Can you work these out from the model? Positions are in its coordinate system, mm. A direction names the side the tool comes from. Give positions to 0.01 mm unless a question says otherwise; leave off trailing zeros. Write each loop counter-clockwise with the first axis right and the second up, starting at its lowest first coordinate (ties: lowest second). Pieces come first, ordered by that corner, then holes.
from build123d import *

# Parameters (mm, degrees)
F0_R     = 1.5
F1_DEPTH = 3
F2_R     = 4.5
F3_DEPTH = 5.2
F4_R     = 1.5
F5_DEPTH = 20


with BuildPart() as f1:
    # F0 (on Front) → F1 (new body)
    with BuildSketch(Plane.XZ):
        with BuildLine():
            Line((5.9394528039, 2.640625), (2.9697264019, 9.3203125))
            ThreePointArc((2.9697264019, 9.3203125), (0, 11.25), (-2.9697264019, 9.3203125))
            Line((-2.9697264019, 9.3203125), (-5.9394528039, 2.640625))
            ThreePointArc((-5.9394528039, 2.640625), (0, -6.5), (5.9394528039, 2.640625))
        make_face()
        with Locations((0, 8)):
            Circle(F0_R, mode=Mode.SUBTRACT)
    extrude(amount=-F1_DEPTH)

    # F2 (on face) → F3 (join)
    with BuildSketch(Plane.XZ):
        Circle(F2_R)
    extrude(amount=F3_DEPTH)

    # F4 (on face) → F5 (cut)
    with BuildSketch(Plane.XZ.offset(5.2)):
        Circle(F4_R)
    extrude(amount=-F5_DEPTH, mode=Mode.SUBTRACT)


solid = f1.part
(1) Will these pins go through, and if not, where does the flat tip stop? P1, Ø2, axis at x = 2.5, y = -0.5, coming from the -Z side; P2, Ø3, axis at y = -2.5, z = 7, coming from the +X side (1 decimal); P3, Ø3, axis at y = 0, z = -1.5, coming from the -X side; P4, Ø3, axis at x = 3, y = 2, coming from the +Z side.
Returned:
P1: stops at z = -6.29
P2: passes through
P3: stops at x = -6.5
P4: stops at z = 10.88
(2) Imagine slicing it at B-B, the plane x = 0. Write out the boundary of the cut face in (y, z), plus the area to 4 significant figures.
Returned:
outline: (-5.2, -4.5) - (0, -4.5) - (0, -6.5) - (3, -6.5) - (3, -1.5) - (-5.2, -1.5) - close; (-5.2, 1.5) - (3, 1.5) - (3, 6.5) - (0, 6.5) - (0, 4.5) - (-5.2, 4.5) - close; (0, 9.5) - (3, 9.5) - (3, 11.25) - (0, 11.25) - close
area: 66.45 mm2
(3) Imagine slicing it at D-D, the plane x = 3.75. Write out the boundary of the cut face in (y, z).
Returned:
outline: (-5.2, -2.49) - (0, -2.49) - (0, -5.31) - (3, -5.31) - (3, 7.57) - (0, 7.57) - (0, 2.49) - (-5.2, 2.49) - close
(4) If I drill on L1, parallel to Z at x = 0, y = 0.9; L2, parallel to Z at x = 0, y = -3.25; L3, parallel to Y at x = -3.75, z = 7.25, over which ranges is the centre line in solid material (lowest first)?
Returned:
L1: z = -6.5 to -1.5, 1.5 to 6.5, 9.5 to 11.25
L2: z = -4.5 to -1.5, 1.5 to 4.5
L3: y = 0 to 3
(5) Imagine slicing it at A-A, the plane z = 0. Write out the boundary of the cut face in (x, y).
Returned:
outline: (-6.5, 0) - (-4.5, 0) - (-4.5, -5.2) - (-1.5, -5.2) - (-1.5, 3) - (-6.5, 3) - close; (1.5, -5.2) - (4.5, -5.2) - (4.5, 0) - (6.5, 0) - (6.5, 3) - (1.5, 3) - close
(6) Imagine slicing it at C-C, the plane y = 0.5. Write out the boundary of the cut face in (x, z).
Returned:
outline: (-5.94, 2.64) arc R6.5 ccw (long way) to (5.94, 2.64) - (2.97, 9.32) arc R3.25 ccw to (-2.97, 9.32) - close; hole circle Ø3 at (0, 0); hole circle Ø3 at (0, 8)
(7) For faces 4 (the face through (-0.59, -2.56, 4.46)), 5 (the face through (-4.434, 1.479, 6.027)), which set-ups out of +Z, -Z, +X, -X, +Y, -Y let a thin tool reach every point of the face, with its end or its side?
Returned:
face 4: -Y
face 5: +Z, -X, +Y, -Y
(8) If we mould it in two halves opening along Z, with no side actions, what happens to faces 1 (the face through (-0.325, 1.479, 6.536)), 2 (the face through (-1.5, 0, 4.5)), 3 (the face through (0.05, 1.48, 11.25))? For each: +Z half, -Z half, draft (parallel to the pull), parting line (faces both ways), or undercut.
Returned:
face 1: undercut
face 2: draft
face 3: +Z half
